Design review of the part shown in the three views and the two pictorial views. Dimensions are in mm from the part's minimum x, y and z. A direction names the side the tool comes from. Round coordinates to 2 decimals unless told otherwise and drop trailing zeros. Loops run counter-clockwise (first coordinate to the right, second up) from the corner with the lowest first, then second, coordinate; pieces in that order, holes last. Notation, with made-up numbers: M -27,77 L 32,77 A21 cw 32,91 Z; hole C 18,14 d3. An arc over 180 degrees is marked long. Answer as CSV lines item,"result". Start each with the question number.
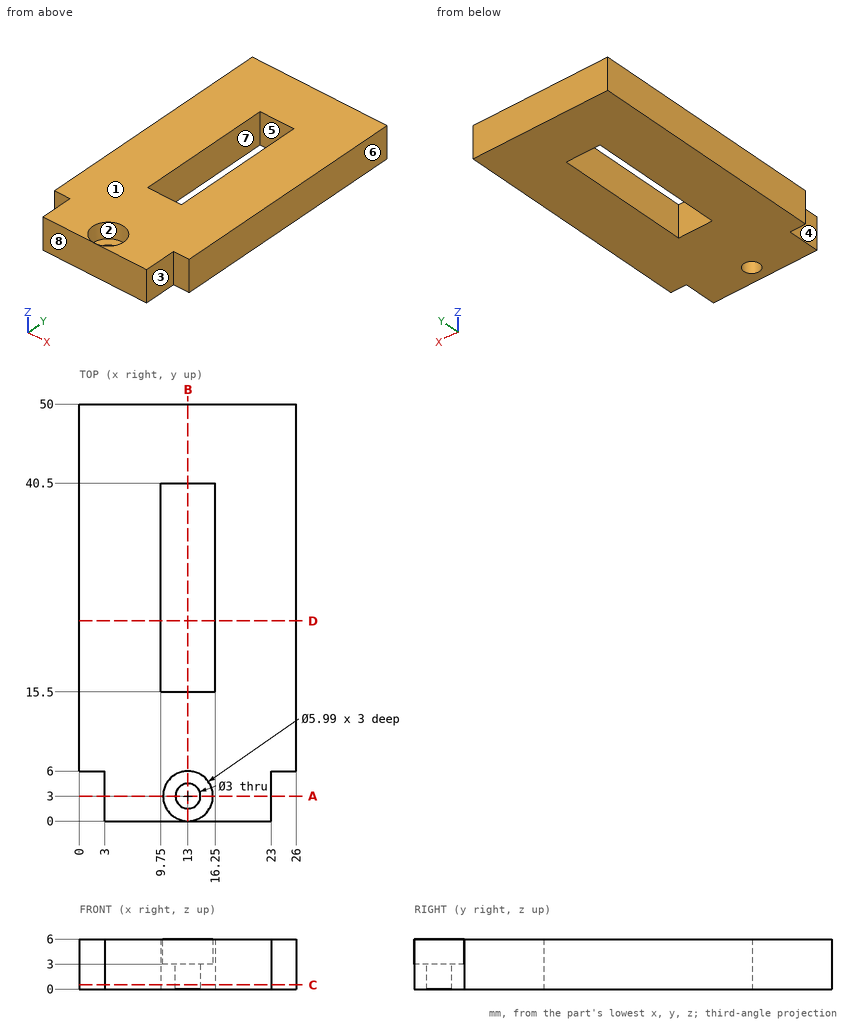
Item 1: Consider section C-C, the plane z = 0.5. Write out the cut boundary in (x, y).
Item 2: Insertion check: pin 1 Ø2 at (x, z) = (9, 5) entering from -Y; pin 2 Ø3 at (x, y) = (13.5, 3.5) entering from +Z; pin 3 Ø3 at (y, z) = (2.5, 3.5) entering from +X; pin 4 Ø1.8 at (y, z) = (1.5, 3) entering from -X. Each pin has a flat end and moves straight along its axis. Give the tip position at first contact, or say it passes through.
Item 3: To check wall thickness, follow line 1 (Y direction, x = 13, z = 2); line 2 (X direction, y = 37, z = 0.95); line 3 (Y direction, x = 15, z = 5.45). State the ranges of each line that lie inside material, in increasing order.
Item 4: The part is to be moulded in two halves that separate along Y. For the marked faces 6, 7 and 8, say which applies: +Y half, -Y half, draft (parallel to the pull), parting line (faces both ways), or undercut.
Item 5: Tool access review of the marked faces 1, 2, 3, 4 and 5: name each direction out of +Z, -Z, +X, -X, +Y, -Y from which nothing blocks a thin tool from reaching the whole face with its end or side.
Item 6: Consider section D-D, the plane y = 24. Write out the cut boundary in (x, z).
Item 7: Consider section A-A, the plane y = 3. Write out the cut boundary in (x, z) (3 decimals).
Item 8: Consider section B-B, the plane x = 13. Write out the cut boundary in (y, z) (3 decimals), then the cut area to 3 significant figures.
Found:
1,outline,"M 0,6 L 3,6 L 3,0 L 23,0 L 23,6 L 26,6 L 26,50 L 0,50 Z; hole M 9.75,15.5 L 16.25,15.5 L 16.25,40.5 L 9.75,40.5 Z; hole C 13,3 d3"
2,pin 1,"stops at y = 0"
2,pin 2,"stops at z = 3"
2,pin 3,"stops at x = 23"
2,pin 4,"stops at x = 3"
3,line 1,"y = 0 to 1.5, 4.5 to 15.5, 40.5 to 50"
3,line 2,"x = 0 to 9.75, 16.25 to 26"
3,line 3,"y = 0 to 0.77, 5.23 to 15.5, 40.5 to 50"
4,face 6,"draft"
4,face 7,"undercut"
4,face 8,"-Y half"
5,face 1,"+Z, +X, -X, +Y, -Y"
5,face 2,"+Z"
5,face 3,"+Z, -Z, +X, -Y"
5,face 4,"+Z, -Z, -X, -Y"
5,face 5,"+Z, -Z"
6,outline,"M 0,0 L 9.75,0 L 9.75,6 L 0,6 Z; M 16.25,0 L 26,0 L 26,6 L 16.25,6 Z"
7,outline,"M 3,0 L 11.5,0 L 11.5,3 L 10.005,3 L 10.005,6 L 3,6 Z; M 14.5,0 L 23,0 L 23,6 L 15.995,6 L 15.995,3 L 14.5,3 Z"
8,outline,"M 0,0 L 1.5,0 L 1.5,3 L 0.005,3 L 0.005,6 L 0,6 Z; M 4.5,0 L 15.5,0 L 15.5,6 L 5.995,6 L 5.995,3 L 4.5,3 Z; M 40.5,0 L 50,0 L 50,6 L 40.5,6 Z"
8,area,"123 mm^2"
